For this review, take the finished solid that the model builds, in its own axes (mm). Face numbers are marked on the shaded views. Give positions to 0.01 mm unless a question says otherwise; leave off trailing zeros. Loops run counter-clockwise (first coordinate to the right, second up) from the corner with the lowest first, then second, coordinate; pieces in that order, holes last. Notation, with made-up numbers: (23.25, -32.75) -> (70.25, -32.75) arc R25 cw to (70.25, -15.75) -> close; hole circle Ø6 at (70, -19.75). An arc over 180 degrees is marked (long way). Answer as CSV lines item,"result". Start each with the question number.
Item 1: The part is to be moulded in two halves that separate along Z. For the marked faces 1, 2 and 3, say which applies: +Z half, -Z half, draft (parallel to the pull), parting line (faces both ways), or undercut.
Item 2: For L1, parallel to Z at x = 5, y = -1.25; L2, parallel to Y at x = 11.5, z = 24.5; L3, parallel to Z at x = 12.5, y = -1.4, list the stretches that pass through material, from the lowest coordinate up. Write a range as from..to.
Item 3: Add section A-A on x = 10.2. State how many separate pieces and enclosed holes the cut face has, plus the area to 3 significant figures.
Item 4: Add section C-C on x = 20. State the section outline as (y, z) points.
Item 5: Clearance check with flat-ended pins moving along their axes: P1, Ø2, axis at x = 18, z = 11.5, coming from the +Y side; P2, Ø1, axis at x = 16.6, z = 25.75, coming from the -Y side; P3, Ø2, axis at x = 20.5, y = -1, coming from the +Z side; P4, Ø2, axis at y = -3.5, z = 13.5, coming from the +X side. State where each tip first meets the part, or that it passes through.
Item 6: Add section B-B on y = -1.7. State the section outline as (x, z) points (3 decimals), plus the area to 3 significant figures.
Item 7: Add section D-D on x = 24. State the section outline as (y, z) points.
```python
from build123d import *

# Parameters (mm, degrees)
F1_DEPTH = 5
F3_DEPTH = 2.5
F5_D     = 3.5
F6_D     = 1.6
F7_D     = 2


with BuildPart() as f1:
    # F0 (on Front) → F1 (new body)
    with BuildSketch(Plane.XZ):
        Polygon((32.376328, 43.667438), (0, 46.5), (0, 0), (39.349691, 3.442652), align=None)
    extrude(amount=F1_DEPTH)

    # F2 (on face) → F3 (cut)
    with BuildSketch(Plane(origin=(0, 0, 0), x_dir=(-1, 0, 0), z_dir=(0, 1, 0))):
        Polygon((-3, 40.214615), (-30.344903, 37.822246), (-35.321901, 9.113185), (-3, 6.285385), align=None)
    extrude(amount=-F3_DEPTH, mode=Mode.SUBTRACT)

    # F5 (through all)
    with Locations(Plane.XZ.offset(5)):
        with Locations((20, 4.399773), (20, 42.100227)):
            Hole(F5_D / 2)

    # F6 (through all)
    with Locations(Plane.XZ.offset(5)):
        with Locations((3.8, 7.75), (3.8, 12.75), (3.8, 20.75), (3.8, 25.75), (3.8, 33.75), (3.8, 38.75), (16.6, 38.75), (16.6, 33.75), (16.6, 25.75), (16.6, 20.75), (16.6, 12.75), (16.6, 7.75)):
            Hole(F6_D / 2)

    # F7 (through all)
    with Locations(Plane.XZ.offset(5)):
        with Locations((10.2, 5.775), (10.2, 14.725), (10.2, 18.775), (10.2, 27.725), (10.2, 31.775), (10.2, 40.725)):
            Hole(F7_D / 2)


solid = f1.part
```
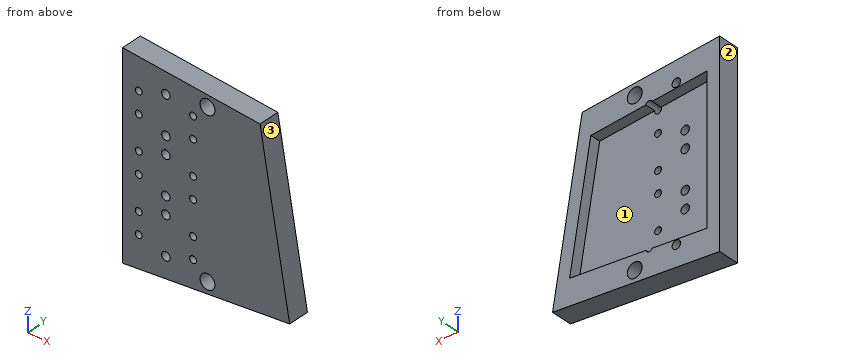
Computed values:
1,face 1,"undercut"
1,face 2,"draft"
1,face 3,"+Z half"
2,L1,"0.44..6.46, 40.04..46.06"
2,L2,"-5..-2.5"
2,L3,"1.09..7.12, 39.38..45.41"
3,separate pieces,"7"
3,enclosed holes,"0"
3,area,"102 mm²"
4,outline,"(-5, 1.75) -> (0, 1.75) -> (0, 2.65) -> (-5, 2.65) -> close; (-5, 6.15) -> (0, 6.15) -> (0, 7.77) -> (-2.5, 7.77) -> (-2.5, 38.73) -> (0, 38.73) -> (0, 40.35) -> (-5, 40.35) -> close; (-5, 43.85) -> (0, 43.85) -> (0, 44.75) -> (-5, 44.75) -> close"
5,P1,"y = -2.5"
5,P2,"through"
5,P3,"z = 44.79"
5,P4,"x = 37.78"
6,outline,"(0, 0) -> (39.35, 3.443) -> (32.376, 43.667) -> (0, 46.5) -> close; hole (3, 6.285) -> (15.875, 7.412) arc R0.8 ccw to (17.373, 7.543) -> (35.322, 9.113) -> (30.345, 37.822) -> (17.373, 38.957) arc R0.8 ccw to (15.875, 39.088) -> (3, 40.215) -> close; hole circle Ø2 at (10.2, 5.775); hole circle Ø2 at (10.2, 40.725); hole circle Ø3.5 at (20, 4.4); hole circle Ø3.5 at (20, 42.1)"
6,area,"595 mm²"
7,outline,"(-5, 2.1) -> (0, 2.1) -> (0, 8.12) -> (-2.5, 8.12) -> (-2.5, 38.38) -> (0, 38.38) -> (0, 44.4) -> (-5, 44.4) -> close"
